Input: part model. Units: mm. Frame: model coordinates. Face numbers are marked on the shaded views. A direction names the side the tool comes from. Give positions to 0.01 mm unless a question says otherwise; leave off trailing zeros. Loops run counter-clockwise (first coordinate to the right, second up) from the corner with the lowest first, then second, coordinate; pieces in that order, holes last. Notation, with made-up numbers: (-32, -27) -> (17, -27) arc R16 ccw to (17, 1) -> close; hole circle Ø11 at (-28, 57.5). An arc over 180 degrees is marked (long way). One line per question, with ' | ' between items.
from build123d import *

# Parameters (mm, degrees)
SKETCH1_W               = 15
SKETCH1_H               = 3.5
BOSS_EXTRUDE1_DEPTH     = 10
CUT_EXTRUDE1_DEPTH      = 13.980754986
CUT_EXTRUDE1_DEPTH_BACK = 13.980754986
FILLET1_R               = 2
SKETCH3_W               = 2.5
SKETCH3_H               = 2.5
CUT_EXTRUDE2_DEPTH      = 8


with BuildPart() as part:
    # Sketch1 → Boss-Extrude1 (new body)
    with BuildSketch(Plane(origin=(0, 0, 0), x_dir=(1, 0, 0), z_dir=(0, 1, 0))):
        Rectangle(SKETCH1_W, SKETCH1_H)
    extrude(amount=BOSS_EXTRUDE1_DEPTH)

    # Sketch2 → Cut-Extrude1 (cut, two sides: drawn at the far end of the back side and taken through both)
    with BuildSketch(Plane.XY.offset(1.75).offset(-CUT_EXTRUDE1_DEPTH_BACK)):
        Polygon((-42.036351416, -19.295421035), (-7.5, 8.063187399), (-5.0550496, 10), (5.0550496, 10), (7.5, 8.063187399), (42.036351416, -19.295421035), (42.036351416, 68.823885013), (-42.036351416, 68.823885013), align=None)
    extrude(amount=CUT_EXTRUDE1_DEPTH + CUT_EXTRUDE1_DEPTH_BACK, mode=Mode.SUBTRACT)

    # Fillet1
    fillet1_edges = [part.edges().sort_by_distance(p)[0] for p in [
        (5.0550496, 10, 0),
        (-5.0550496, 10, 0),
    ]]
    fillet(fillet1_edges, radius=FILLET1_R)

    # Sketch3 → Cut-Extrude2 (cut)
    with BuildSketch(Plane(origin=(0, 10, 0), x_dir=(1, 0, 0), z_dir=(0, 1, 0))):
        with Locations((-1.875, 0)):
            Rectangle(SKETCH3_W, SKETCH3_H)
        with Locations((-5.625, 0)):
            Rectangle(SKETCH3_W, SKETCH3_H)
        with Locations((5.625, 0)):
            Rectangle(SKETCH3_W, SKETCH3_H)
        with Locations((1.875, 0)):
            Rectangle(SKETCH3_W, SKETCH3_H)
    extrude(amount=-CUT_EXTRUDE2_DEPTH, mode=Mode.SUBTRACT)


solid = part.part
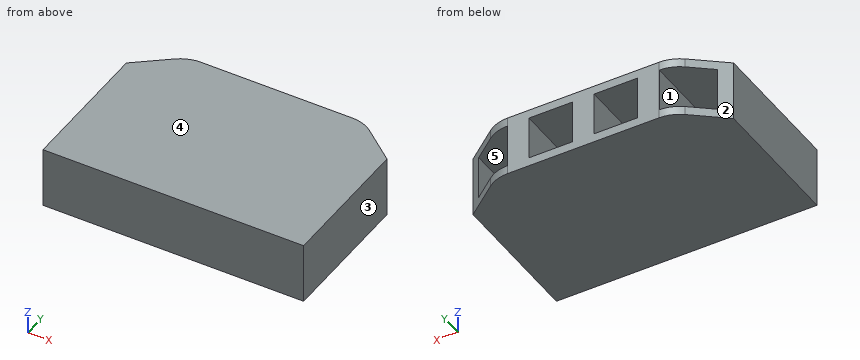
1. Section query B-B (z = 1.55). Output: boundary loops of the cut face in (x, y), then the cut area to 3 significant figures.
Determined:
outline: (-7.5, 0) -> (7.5, 0) -> (7.5, 8.06) -> (5.6, 9.57) arc R2 ccw to (4.36, 10) -> (-4.36, 10) arc R2 ccw to (-5.6, 9.57) -> (-7.5, 8.06) -> close | area: 145 mm2
2. Section query C-C (y = 5.5). Output: boundary loops of the cut face in (x, z) (3 decimals), then the cut area to 3 significant figures.
Determined:
outline: (-7.5, -1.75) -> (7.5, -1.75) -> (7.5, 1.75) -> (-7.5, 1.75) -> close; hole (-6.875, -1.25) -> (-4.375, -1.25) -> (-4.375, 1.25) -> (-6.875, 1.25) -> close; hole (-3.125, -1.25) -> (-0.625, -1.25) -> (-0.625, 1.25) -> (-3.125, 1.25) -> close; hole (0.625, -1.25) -> (3.125, -1.25) -> (3.125, 1.25) -> (0.625, 1.25) -> close; hole (4.375, -1.25) -> (6.875, -1.25) -> (6.875, 1.25) -> (4.375, 1.25) -> close | area: 27.5 mm2
3. Section query A-A (x = 1). Output: boundary loops of the cut face in (y, z), then the cut area to 3 significant figures.
Determined:
outline: (0, -1.75) -> (10, -1.75) -> (10, -1.25) -> (2, -1.25) -> (2, 1.25) -> (10, 1.25) -> (10, 1.75) -> (0, 1.75) -> close | area: 15.0 mm2
4. Pull-direction query (X, two-part tool) for the marked faces 3, 4 and 5; classes: pulls with the +X half, pulls with the -X half, needs draft (parallel to the pull), parting line crosses it, or undercut.
Determined:
face 3: pulls with the +X half | face 4: needs draft | face 5: undercut
5. Reachability of the marked faces 1 and 2 from +Z, -Z, +X, -X, +Y, -Y: full face, straight path, thin tool, end or side. Return the list, or none.
Determined:
face 1: +Y | face 2: +Z, -Z, -X, +Y
6. Ray query, line 1 along X through (y, z) = (6, -0.7) (3 decimals); line 2 along X through (y, z) = (9.25, 0.1) (3 decimals); line 3 along Z through (x, y) = (-3, 8.25). Return the intervals inside material, ascending. Write a range as from..to.
Determined:
line 1: x = -7.5..-6.875, -4.375..-3.125, -0.625..0.625, 3.125..4.375, 6.875..7.5 | line 2: x = -4.375..-3.125, -0.625..0.625, 3.125..4.375 | line 3: z = -1.75..-1.25, 1.25..1.75
7. Pin query (flat end, axial travel): P1, Ø1.2, axis at x = -2, z = 0, coming from the +Y side; P2, Ø2, axis at x = -5, z = 0.5, coming from the +Y side. Return the tip coordinate at first contact, or that it passes through.
Determined:
P1: stops at y = 2 | P2: stops at y = 10
